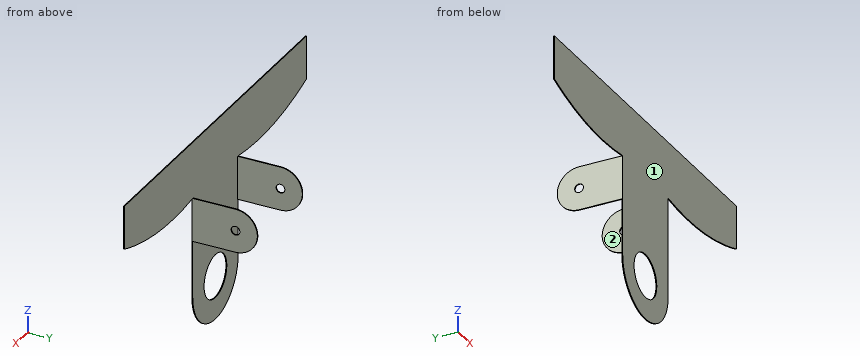
```python
from build123d import *

# Parameters (mm, degrees)
SKETCH_1_R      = 5
EXTRUDE_1_DEPTH = 0.1
SKETCH_3_R      = 1
EXTRUDE_2_DEPTH = 0.2
SKETCH_4_R      = 1
EXTRUDE_3_DEPTH = 0.2


with BuildPart() as part:
    # 草图1 → 凸台-拉伸1 (new body, symmetric)
    with BuildSketch(Plane(origin=(0, 0, 0), x_dir=(1, 0, 0), z_dir=(0, 1, 0))):
        with BuildLine():
            Line((10, 0), (10, -23))
            add(Edge.make_bspline(
                [(10, -23), (25.285299712, -20.780872621), (40, -26)],
                knots=[0, 0, 0, 1, 1, 1], degree=2))
            Line((40, -26), (40, -36))
            Line((40, -36), (-40, -36))
            Line((-40, -36), (-40, -26))
            add(Edge.make_bspline(
                [(-10, -23), (-25.285299712, -20.780872621), (-40, -26)],
                knots=[0, 0, 0, 1, 1, 1], degree=2))
            Line((-10, -23), (-10, 0))
            ThreePointArc((-10, 0), (0, 10), (10, 0))
        make_face()
        Circle(SKETCH_1_R, mode=Mode.SUBTRACT)
    extrude(amount=EXTRUDE_1_DEPTH, both=True)

    # 草图3 → 凸台-拉伸2 (add)
    with BuildSketch(Plane(origin=(10, 0, 0), x_dir=(0, 0, -1), z_dir=(1, 0, 0))):
        with BuildLine():
            Line((-23, -0.1), (-13, -0.1))
            Line((-13, -0.1), (-13, 9.9))
            ThreePointArc((-13, 9.9), (-18, 14.9), (-23, 9.9))
            Line((-23, 9.9), (-23, -0.1))
        make_face()
        with Locations((-18, 9.9)):
            Circle(SKETCH_3_R, mode=Mode.SUBTRACT)
    extrude(amount=-EXTRUDE_2_DEPTH)

    # 草图4 → 凸台-拉伸3 (add)
    with BuildSketch(Plane.ZY.offset(10)):
        with BuildLine():
            Line((23, -0.1), (13, -0.1))
            Line((13, -0.1), (13, 9.9))
            ThreePointArc((13, 9.9), (18, 14.9), (23, 9.9))
            Line((23, 9.9), (23, -0.1))
        make_face()
        with Locations((18, 9.9)):
            Circle(SKETCH_4_R, mode=Mode.SUBTRACT)
    extrude(amount=-EXTRUDE_3_DEPTH)


solid = part.part
```
Part model, mm, in its own coordinate system. Face numbers are marked on the shaded views. A direction names the side the tool comes from. Round coordinates to 2 decimals unless told otherwise and drop trailing zeros. Write each loop counter-clockwise with the first axis right and the second up, starting at its lowest first coordinate (ties: lowest second). Pieces come first, ordered by that corner, then holes.
Item 1: Probe L1, parallel to X at y = 0, z = 0; L2, parallel to Z at x = 0, y = 0.05; L3, parallel to Y at x = -9.9, z = 18. List the from-to ranges inside material, lowest first.
Results:
L1: x = -10 to -5, 5 to 10
L2: z = -10 to -5, 5 to 36
L3: y = -0.1 to 8.9, 10.9 to 14.9
Item 2: Cut at A-A, the plane z = 18. Give the cut face in (x, y).
Results:
outline: (-10, -0.1) - (10, -0.1) - (10, 8.9) - (9.8, 8.9) - (9.8, 0.1) - (-9.8, 0.1) - (-9.8, 8.9) - (-10, 8.9) - close; (-10, 10.9) - (-9.8, 10.9) - (-9.8, 14.9) - (-10, 14.9) - close; (9.8, 10.9) - (10, 10.9) - (10, 14.9) - (9.8, 14.9) - close
Item 3: Cut at C-C, the plane x = 0. Give the cut face in (y, z).
Results:
outline: (-0.1, -10) - (0.1, -10) - (0.1, -5) - (-0.1, -5) - close; (-0.1, 5) - (0.1, 5) - (0.1, 36) - (-0.1, 36) - close
Item 4: Which spindle directions (+Z, -Z, +X, -X, +Y, -Y) get a long thin tool onto all of the face, cutting with end or side? Do the marked faces 1 and 2. Say none if no direction does.
Results:
face 1: +Z, -Z, +X, -X, -Y
face 2: +Z, -Z, +Y
Item 5: Cut at B-B, the plane y = 3.75. Give the cut face in (x, z), plus the area to 3 significant figures.
Results:
outline: (-10, 13) - (-9.8, 13) - (-9.8, 23) - (-10, 23) - close; (9.8, 13) - (10, 13) - (10, 23) - (9.8, 23) - close
area: 4.00 mm2
Item 6: Drop flat-ended pins along their axis: pin 1 Ø3 at (y, z) = (5.5, 14) entering from -X; pin 2 Ø8 at (y, z) = (7.5, 20) entering from +X; pin 3 Ø13 at (x, z) = (0, 0) entering from +Y. Give the stop position or say it passes through.
Results:
pin 1: stops at x = -10
pin 2: stops at x = 10
pin 3: stops at y = 0.1
